Check sheet for the modelled part. Datum: model origin and axes. Units: mm. Face numbers are marked on the shaded views. A direction names the side the tool comes from. Round coordinates to 2 decimals unless told otherwise and drop trailing zeros. Loops run counter-clockwise (first coordinate to the right, second up) from the corner with the lowest first, then second, coordinate; pieces in that order, holes last. Notation, with made-up numbers: (60.25, 34) -> (69.25, 34) arc R29 cw to (69.25, 66) -> close; hole circle Ø8 at (54, 49.5). An arc over 180 degrees is marked (long way). Return JSON: item names as keys, results as strings.
Autodesk Inventor part; units mm, degrees
ref_plane "YZ Plane" through (0, 0, 0) normal (1, 0, 0) x (0, 1, 0)
ref_plane "XZ Plane" through (0, 0, 0) normal (0, 1, 0) x (-1, 0, 0)
ref_plane "XY Plane" through (0, 0, 0) normal (0, 0, 1) x (1, 0, 0)
sketch "Esquisse1" plane through (0, 0, 0) normal (0, 1, 0) x (-1, 0, 0)
  line L0 (89.3861, -273.097) -> (89.3861, -280.097)
  line L1 (89.3861, -250.597) -> (89.3861, -263.7609)
  line L2 (89.3861, -302.597) -> (79.3861, -302.597)
  line L3 (79.3861, -302.597) -> (79.3861, -250.597)
  line L4 (122.5932, -263.7609) -> (89.3861, -263.7609)
  line L5 (89.3861, -268.7609) -> (122.5932, -268.7609)
  line L6 (122.5932, -289.4332) -> (89.3861, -289.4332)
  line L7 (89.3861, -284.4332) -> (122.5932, -284.4332)
  line L8 (89.3861, -289.4332) -> (89.3861, -302.597)
  line L9 (89.3861, -268.7609) -> (89.3861, -284.4332)
  line L10 (79.3861, -250.597) -> (89.3861, -250.597)
  line L11 (122.5932, -263.7609) -> (122.5932, -268.7609)
  line L12 (122.5932, -284.4332) -> (122.5932, -289.4332)
  point P0 (0, 0)
  dimension "d0" = 10
  dimension "d1" = 5
  dimension "d2" = 5
extrude "Extrusion1" add sketch "Esquisse1" along normal blind 15
properties part number "haut support"
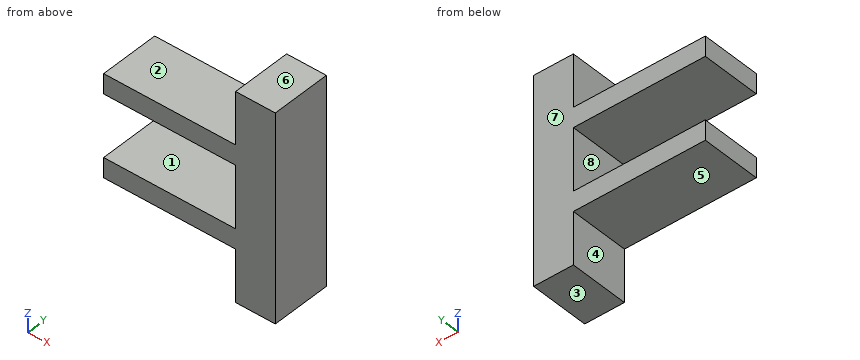
Q1. Material ranges on line 1 (Z direction, x = -109, y = 1); line 2 (X direction, y = 4.75, z = -260), recorded low to high.
Results list:
{"line 1": "-289.43 to -284.43, -268.76 to -263.76", "line 2": "-89.39 to -79.39"}
Q2. Section check B-B (y = 2.5). Record the boundary of the cut face in (x, z).
Results list:
{"outline": "(-122.59, -289.43) -> (-89.39, -289.43) -> (-89.39, -302.6) -> (-79.39, -302.6) -> (-79.39, -250.6) -> (-89.39, -250.6) -> (-89.39, -263.76) -> (-122.59, -263.76) -> (-122.59, -268.76) -> (-89.39, -268.76) -> (-89.39, -284.43) -> (-122.59, -284.43) -> close"}
Q3. Draft check along Z on the marked faces 5, 6, 7 and 8. Enter one of: released by +Z, released by -Z, zero draft, split by the parting line, or undercut.
Results list:
{"face 5": "released by -Z", "face 6": "released by +Z", "face 7": "zero draft", "face 8": "undercut"}
Q4. Go/stop test with flat-tipped pins: pin 1 (4.5 mm diameter, centred on x = -103.5, y = 7, fed in from -Z); pin 2 (6.5 mm diameter, centred on y = 5.5, z = -260, fed in from -X); pin 3 (7.5 mm diameter, centred on x = -106, y = 9, fed in from +Z). Record where each tip stops, or that it passes through.
Results list:
{"pin 1": "z = -289.43", "pin 2": "x = -89.39", "pin 3": "z = -263.76"}
Q5. Tool access check on the marked faces 1, 2, 3 and 4. Record the directions out of +Z, -Z, +X, -X, +Y, -Y that give a thin tool (end or side, any length) a straight path to the whole face; none if there is none.
Results list:
{"face 1": "-X, +Y, -Y", "face 2": "+Z, -X, +Y, -Y", "face 3": "-Z, +X, -X, +Y, -Y", "face 4": "-Z, -X, +Y, -Y"}
Q6. Section check C-C (z = -277.5). Record the boundary of the cut face in (x, y).
Results list:
{"outline": "(-89.39, 0) -> (-79.39, 0) -> (-79.39, 15) -> (-89.39, 15) -> close"}
Q7. Section check A-A (x = -110). Record the boundary of the cut face in (y, z).
Results list:
{"outline": "(0, -289.43) -> (15, -289.43) -> (15, -284.43) -> (0, -284.43) -> close; (0, -268.76) -> (15, -268.76) -> (15, -263.76) -> (0, -263.76) -> close"}
